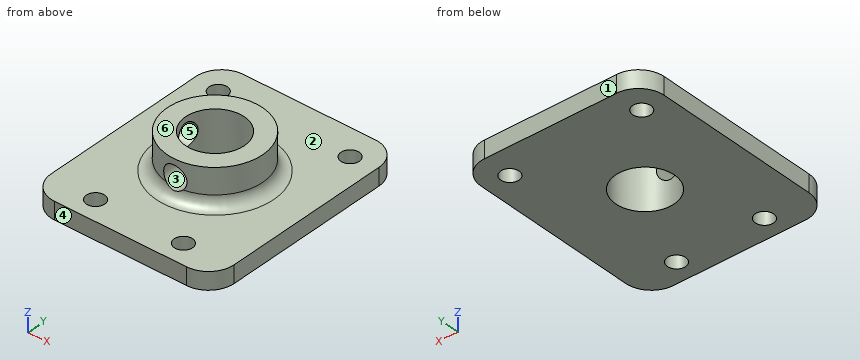
from build123d import *

# Parameters (mm, degrees)
CROQUIS1_W              = 50
CROQUIS1_H              = 60
SALIENTE_EXTRUIR1_DEPTH = 4.7625
CROQUIS2_R              = 13
SALIENTE_EXTRUIR2_DEPTH = 10
CROQUIS3_R              = 8
CORTAR_EXTRUIR1_DEPTH   = 42.748429985
CROQUIS4_R              = 2.5
CORTAR_EXTRUIR2_DEPTH   = 41.311288741
REDONDEO1_R             = 3
REDONDEO2_R             = 7
CROQUIS5_R              = 3.175
CORTAR_EXTRUIR3_DEPTH   = 42.748429985
CROQUIS6_R              = 3.175
CORTAR_EXTRUIR4_DEPTH   = 42.748430021


with BuildPart() as part:
    # Croquis1 → Saliente-Extruir1 (new body)
    with BuildSketch(Plane.XY):
        Rectangle(CROQUIS1_W, CROQUIS1_H)
    extrude(amount=SALIENTE_EXTRUIR1_DEPTH)

    # Croquis2 → Saliente-Extruir2 (add)
    with BuildSketch(Plane.XY.offset(4.7625)):
        Circle(CROQUIS2_R)
    extrude(amount=SALIENTE_EXTRUIR2_DEPTH)

    # Croquis3 → Cortar-Extruir1 (cut, through all)
    with BuildSketch(Plane.XY.offset(14.7625)):
        Circle(CROQUIS3_R)
    extrude(amount=-CORTAR_EXTRUIR1_DEPTH, mode=Mode.SUBTRACT)

    # Croquis4 → Cortar-Extruir2 (cut, through all)
    with BuildSketch(Plane.XY.offset(4.7625)):
        with Locations((18, 22)):
            Circle(CROQUIS4_R)
        with Locations((12, -24)):
            Circle(CROQUIS4_R)
        with Locations((-12, -24)):
            Circle(CROQUIS4_R)
        with Locations((-18, 22)):
            Circle(CROQUIS4_R)
    extrude(amount=-CORTAR_EXTRUIR2_DEPTH, mode=Mode.SUBTRACT)

    # Redondeo1
    redondeo1_edges = [part.edges().sort_by_distance(p)[0] for p in [
        (-13, 0, 4.7625),
    ]]
    fillet(redondeo1_edges, radius=REDONDEO1_R)

    # Redondeo2
    redondeo2_edges = [part.edges().sort_by_distance(p)[0] for p in [
        (25, -30, 2.38125),
        (-25, -30, 2.38125),
        (-25, 30, 2.38125),
        (25, 30, 2.38125),
    ]]
    fillet(redondeo2_edges, radius=REDONDEO2_R)

    # Croquis5 → Cortar-Extruir3 (cut, through all)
    with BuildSketch(Plane(origin=(0, 0, 0), x_dir=(1, 0, 0), z_dir=(0, 1, 0))):
        with Locations(Location((0, -10, 0), (0, 0, 270))):
            Circle(CROQUIS5_R)
    extrude(amount=-CORTAR_EXTRUIR3_DEPTH, mode=Mode.SUBTRACT)

    # Croquis6 → Cortar-Extruir4 (cut, through all)
    with BuildSketch(Plane(origin=(0, 0, 0), x_dir=(0, 0, -1), z_dir=(1, 0, 0))):
        with Locations((-10, 0)):
            Circle(CROQUIS6_R)
    extrude(amount=-CORTAR_EXTRUIR4_DEPTH, mode=Mode.SUBTRACT)


solid = part.part
For this review, take the finished solid that the model builds, in its own axes (mm). Face numbers are marked on the shaded views. A direction names the side the tool comes from. Coordinates: 2 decimals unless noted, no trailing zeros. Order: outer loops, then holes, each group sorted by start corner. A loop starts at its lowest first (then second) coordinate and runs counter-clockwise, first axis right, second up. Notation, with made-up numbers: (27, 69) - (45, 69) arc R20 cw to (45, 97) - close; hole circle Ø3 at (53.5, 34.5). An arc over 180 degrees is marked (long way). Answer as CSV lines item,"result". Start each with the question number.
1) Draft analysis for pull direction Z (two halves, no side actions). For the marked faces 3, 4, 5 and 6, state which applies: +Z half, -Z half, draft (parallel to the pull), parting line (faces both ways), or undercut.
2) To check wall thickness, follow line 1 along Y through (x, z) = (-18, 2.65); line 2 along X through (y, z) = (24, 3.5); line 3 along Z through (x, y) = (-20.5, -23). State the ranges of each line that lie inside material, in increasing order. Write a range as [from, to].
3) Add section D-D (y = 0). State the section outline as (x, z) points (1 decimal).
4) Insertion check: P1, Ø5, axis at y = 0, z = 10, coming from the +X side; P2, Ø2, axis at x = 10.5, z = 12.5, coming from the -Y side; P3, Ø8, axis at x = -12, y = -24, coming from the +Z side. Each pin has a flat end and moves straight along its axis. Give the tip position at first contact, or say it passes through.
5) Add section B-B (x = 0). State the section outline as (y, z) points (1 decimal).
6) Add section A-A (y = 22). State the section outline as (x, z) points, then the cut area to 4 significant figures.
7) Machinability: for the marked faces 1 and 2, which of the approach directions +Z, -Z, +X, -X, +Y, -Y give a long, thin tool a straight path to every point of the face, cutting with its end or side? Answer none if there is none.
8) Add section C-C (z = 10). State the section outline as (x, y) points (3 decimals).
Result:
1,face 3,"undercut"
1,face 4,"draft"
1,face 5,"undercut"
1,face 6,"+Z half"
2,line 1,"[-30, 19.5], [24.5, 30]"
2,line 2,"[-24.93, -19.5], [-16.5, 16.5], [19.5, 24.93]"
2,line 3,"[0, 4.76]"
3,outline,"(-25, 0) - (-8, 0) - (-8, 6.8) - (-13.2, 6.8) arc R3 cw to (-16, 4.8) - (-25, 4.8) - close; (-13, 13.2) - (-8, 13.2) - (-8, 14.8) - (-13, 14.8) - close; (8, 0) - (25, 0) - (25, 4.8) - (16, 4.8) arc R3 cw to (13, 7.8) - (13, 14.8) - (8, 14.8) - close"
4,P1,"x = 13.01"
4,P2,"y = -8.87"
4,P3,"z = 4.76"
5,outline,"(-30, 0) - (-8, 0) - (-8, 6.8) - (-13.2, 6.8) arc R3 cw to (-16, 4.8) - (-30, 4.8) - close; (-13, 13.2) - (-8, 13.2) - (-8, 14.8) - (-13, 14.8) - close; (8, 0) - (30, 0) - (30, 4.8) - (16, 4.8) arc R3 cw to (13, 7.8) - (13, 14.8) - (8, 14.8) - close"
6,outline,"(-25, 0) - (-20.5, 0) - (-20.5, 4.76) - (-25, 4.76) - close; (-15.5, 0) - (15.5, 0) - (15.5, 4.76) - (-15.5, 4.76) - close; (20.5, 0) - (25, 0) - (25, 4.76) - (20.5, 4.76) - close"
6,area,"190.5 mm^2"
7,face 1,"+Z, -Z, +X, -X, +Y"
7,face 2,"+Z"
8,outline,"(-12.606, -3.175) arc R13 ccw to (-3.175, -12.606) - (-3.175, -7.343) arc R8 cw to (-7.343, -3.175) - close; (-12.606, 3.175) - (-7.343, 3.175) arc R8 cw (long way) to (3.175, -7.343) - (3.175, -12.606) arc R13 ccw (long way) to start"
